Check sheet for the modelled part. Datum: model origin and axes. Units: mm. A direction names the side the tool comes from. Coordinates: 2 decimals unless noted, no trailing zeros. Order: outer loops, then holes, each group sorted by start corner. A loop starts at its lowest first (then second) coordinate and runs counter-clockwise, first axis right, second up. Notation, with made-up numbers: M -19.75,-3 L 9.25,-3 A18 ccw 9.25,22 Z; hole C -21.5,14 d1. An arc over 180 degrees is marked long. Answer in a Markdown table with one row per item. Add a question column.
from build123d import *

# Parameters (mm, degrees)
SM_BASE_FLANGE_1_DEPTH = 20
EXTRUDE_1_DEPTH        = 2
EXTRUDE_START          = -2
EXTRUDE_2_DEPTH        = 2
SKETCH_8_R             = 4
SKETCH_8_R_2           = 1.1
CUT_EXTRUDE_1_DEPTH    = 65.618145883
SKETCH_9_R             = 3
SKETCH_9_R_2           = 1.5
CUT_EXTRUDE_2_DEPTH    = 2


# Sheet-metal steps are written as plain solids
with BuildPart() as part:
    # Sketch 1 → 基体-法兰1 (new body)
    with BuildSketch(Plane.XY):
        with BuildLine():
            Line((-12.079491004, 12.945691914), (-12.079491004, -8.117708086))
            ThreePointArc((-12.079491004, -8.117708086), (-11.863745859, -8.638562941), (-11.342891004, -8.854308086))
            Line((-11.342891004, -8.854308086), (40.183908996, -8.854308086))
            ThreePointArc((40.183908996, -8.854308086), (40.704763851, -8.638562941), (40.920508996, -8.117708086))
            Line((40.920508996, -8.117708086), (40.920508996, 12.945691914))
            Line((40.920508996, 12.945691914), (42.920508996, 12.945691914))
            Line((42.920508996, 12.945691914), (42.920508996, -8.117708086))
            ThreePointArc((42.920508996, -8.117708086), (42.118977413, -10.052776503), (40.183908996, -10.854308086))
            Line((40.183908996, -10.854308086), (-11.342891004, -10.854308086))
            ThreePointArc((-11.342891004, -10.854308086), (-13.277959422, -10.052776503), (-14.079491004, -8.117708086))
            Line((-14.079491004, -8.117708086), (-14.079491004, 12.945691914))
            Line((-14.079491004, 12.945691914), (-12.079491004, 12.945691914))
        make_face()
    extrude(amount=SM_BASE_FLANGE_1_DEPTH)

    # 草图6 → 凸台-拉伸1 (add)
    with BuildSketch(Plane.ZY.offset(14.079491004)):
        with BuildLine():
            Line((0, 12.945691914), (20, 12.945691914))
            ThreePointArc((20, 12.945691914), (10, 22.945691914), (0, 12.945691914))
        make_face()
    extrude(amount=-EXTRUDE_1_DEPTH)

    # 草图7 → 凸台-拉伸2 (add)
    with BuildSketch(Plane(origin=(42.920508996, 0, 0), x_dir=(0, 0, -1), z_dir=(1, 0, 0)).offset(EXTRUDE_START)):
        with BuildLine():
            Line((-20, 12.945691914), (0, 12.945691914))
            ThreePointArc((0, 12.945691914), (-10, 22.945691914), (-20, 12.945691914))
        make_face()
    extrude(amount=EXTRUDE_2_DEPTH)

    # 草图8 → 切除-拉伸1 (cut, through all)
    with BuildSketch(Plane.ZY.offset(14.079491004)):
        with Locations((10, 12.945691914)):
            Circle(SKETCH_8_R)
        with Locations((10, 19.945691914)):
            Circle(SKETCH_8_R_2)
        with Locations((17, 12.945691914)):
            Circle(SKETCH_8_R_2)
        with Locations((10, 5.945691914)):
            Circle(SKETCH_8_R_2)
        with Locations((3, 12.945691914)):
            Circle(SKETCH_8_R_2)
    extrude(amount=-CUT_EXTRUDE_1_DEPTH, mode=Mode.SUBTRACT)

    # 草图9 → 切除-拉伸2 (cut)
    with BuildSketch(Plane(origin=(0, -10.854308086, 0), x_dir=(-1, 0, 0), z_dir=(0, -1, 0))):
        with Locations(Location((-14.420508996, -10, 0), (0, 0, 90))):
            Circle(SKETCH_9_R)
        with Locations(Location((-29.370256464, -5.050252532, 0), (0, 0, 90))):
            Circle(SKETCH_9_R_2)
        with Locations(Location((-19.370256464, -5.050252532, 0), (0, 0, 90))):
            Circle(SKETCH_9_R_2)
        with Locations(Location((-9.470761527, -5.050252532, 0), (0, 0, 90))):
            Circle(SKETCH_9_R_2)
        with Locations(Location((-19.370256464, -14.949747468, 0), (0, 0, 90))):
            Circle(SKETCH_9_R_2)
        with Locations(Location((-9.470761527, -14.949747468, 0), (0, 0, 90))):
            Circle(SKETCH_9_R_2)
        with Locations(Location((-29.370256464, -14.949747468, 0), (0, 0, 90))):
            Circle(SKETCH_9_R_2)
        with Locations(Location((0.529238473, -5.050252532, 0), (0, 0, 90))):
            Circle(SKETCH_9_R_2)
        with Locations(Location((0.529238473, -14.949747468, 0), (0, 0, 90))):
            Circle(SKETCH_9_R_2)
    extrude(amount=-CUT_EXTRUDE_2_DEPTH, mode=Mode.SUBTRACT)


solid = part.part
1. Section check C-C on z = 10. State how many separate pieces and enclosed holes the cut face has, then the cut area to 3 significant figures.
2. Scan lines: line 1 (X direction, y = 16, z = 15); line 2 (Y direction, x = -1, z = 1.75); line 3 (Y direction, x = 41.5, z = 10). Record each from-to range of solid material in increasing order.
3. Section check A-A on y = 1. Enter the section's corners in (x, z), then the cut area to 3 significant figures.
4. Release check for a two-part mould opening along Z. For faces 1 (the cylindrical face through (41.907, 22.943, 9.78)), 2 (the flat face through (40.921, 8, 10)), 3 (the cylindrical face through (18.796, -9.868, 13.564)) record: released by +Z, released by -Z, zero draft, split by the parting line, or undercut.
5. Go/stop test with flat-tipped pins: pin 1 Ø10 at (x, z) = (-4, 12.5) entering from +Y; pin 2 Ø2.5 at (x, z) = (19.37, 5.05) entering from -Y. Record where each tip stops, or that it passes through.
6. Set-up check for faces 4 (the flat face through (14, -8.854, 5)), 5 (the cylindrical face through (12.595, -9.868, 12.381)): record each of +Z, -Z, +X, -X, +Y, -Y from which the full face is reachable in a straight line by a thin tool's end or side.
7. Section check B-B on z = 4.75. Enter the section's corners in (x, y), then the cut area to 3 significant figures.
8. Section check D-D on x = 22. Enter the section's corners in (y, z).
Result sheet:
| question | item | result |
|---|---|---|
| 1 | separate pieces | 8 |
| 1 | enclosed holes | 0 |
| 1 | area | 177 mm^2 |
| 2 | line 1 | -14.08 to -12.08, 40.92 to 42.92 |
| 2 | line 2 | -10.85 to -8.85 |
| 2 | line 3 | -10.52 to 4.85, 7.05 to 8.95, 16.95 to 18.85, 21.05 to 22.95 |
| 3 | outline | M -14.08,0 L -12.08,0 L -12.08,20 L -14.08,20 Z; M 40.92,0 L 42.92,0 L 42.92,20 L 40.92,20 Z |
| 3 | area | 80.0 mm^2 |
| 4 | face 1 | split by the parting line |
| 4 | face 2 | zero draft |
| 4 | face 3 | undercut |
| 5 | pin 1 | y = -8.85 |
| 5 | pin 2 | through |
| 6 | face 4 | +Z, -Z, +Y |
| 6 | face 5 | +Y, -Y |
| 7 | outline | M -14.08,-8.12 A2.74 ccw -11.34,-10.85 L -2,-10.85 L -2,-8.85 L -11.34,-8.85 A0.74 cw -12.08,-8.12 L -12.08,21.46 L -14.08,21.46 Z; M 0.94,-10.85 L 8,-10.85 L 8,-8.85 L 0.94,-8.85 Z; M 10.94,-10.85 L 17.9,-10.85 L 17.9,-8.85 L 10.94,-8.85 Z; M 20.84,-10.85 L 27.9,-10.85 L 27.9,-8.85 L 20.84,-8.85 Z; M 30.84,-10.85 L 40.18,-10.85 A2.74 ccw 42.92,-8.12 L 42.92,21.46 L 40.92,21.46 L 40.92,-8.12 A0.74 cw 40.18,-8.85 L 30.84,-8.85 Z |
| 7 | area | 209 mm^2 |
| 8 | outline | M -10.85,0 L -8.85,0 L -8.85,20 L -10.85,20 Z |
